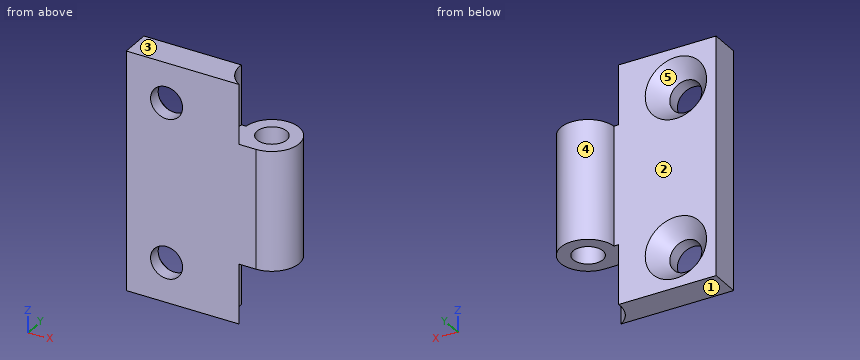
```python
from build123d import *

# Parameters (mm, degrees)
SKETCH1_R                                    = 2.38125
EXTRUDE1_DEPTH                               = 19.05
CUT_EXTRUDE1_DEPTH                           = 9.525
CSK_FOR_10_FLAT_HEAD_MACHINE_SCREW1_AT_COUNT = 2
CSK_FOR_10_FLAT_HEAD_MACHINE_SCREW1_AT_PITCH = 25.4


with BuildPart() as part:
    # Sketch1 → Extrude1 (new, symmetric)
    with BuildSketch(Plane.XY):
        with BuildLine():
            Line((-20.6375, 0), (0, 0))
            ThreePointArc((0, 0), (3.219925902, 1.417615701), (4.348688447, 4.7498))
            ThreePointArc((4.348688447, 4.7498), (0, 8.73125), (-4.348688447, 4.7498))
            Line((-4.348688447, 4.7498), (-20.6375, 4.7498))
            Line((-20.6375, 4.7498), (-20.6375, 0))
        make_face()
        with Locations(Location((0, 4.365625, 0), (0, 0, 180))):
            Circle(SKETCH1_R, mode=Mode.SUBTRACT)
    extrude(amount=EXTRUDE1_DEPTH, both=True)

    # Sketch2 → Cut-Extrude1 (cut)
    with BuildSketch(Plane.XY.offset(19.05)):
        with BuildLine():
            Line((-5.110688447, 4.7498), (-4.348688447, 4.7498))
            ThreePointArc((-4.348688447, 4.7498), (3.936533663, 7.969725902), (0, 0))
            Line((0, 0), (-2.684780288, 0))
            ThreePointArc((-2.684780288, 0), (-4.564261518, 2.034478581), (-5.110688447, 4.7498))
        make_face()
    cut_extrude1 = extrude(amount=-CUT_EXTRUDE1_DEPTH, mode=Mode.SUBTRACT)

    # Mirror1: Cut-Extrude1 across plane
    add(cut_extrude1.mirror(Plane.XY), mode=Mode.SUBTRACT)

    # Sketch6 → CSK for #10 Flat Head Machine Screw1 (revolve, cut)
    with BuildSketch(Plane(origin=(-14.224, 4.7498, -12.7), x_dir=(0, 0, 1), z_dir=(1, 0, 0))):
        Polygon((0, 0), (0, 4.7498), (2.5527, 4.7498), (2.5527, 2.688180894), (4.8895, 0), align=None)
    csk_for_10_flat_head_machine_screw1 = revolve(axis=Axis((-14.224, 11.0998, -12.7), (0, -1, 0)), mode=Mode.SUBTRACT)

    # CSK for #10 Flat Head Machine Screw1 at: CSK for #10 Flat Head Machine Screw1 ×2
    with Locations(*[(0, 0, i * CSK_FOR_10_FLAT_HEAD_MACHINE_SCREW1_AT_PITCH) for i in range(1, CSK_FOR_10_FLAT_HEAD_MACHINE_SCREW1_AT_COUNT)]):
        add(csk_for_10_flat_head_machine_screw1, mode=Mode.SUBTRACT)


solid = part.part
```
Could you check a few things on this model? Use its own coordinates, in mm. Face numbers are marked on the shaded views. A direction names the side the tool comes from. Round coordinates to 2 decimals unless told otherwise and drop trailing zeros. Loops run counter-clockwise (first coordinate to the right, second up) from the corner with the lowest first, then second, coordinate; pieces in that order, holes last. Notation, with made-up numbers: (0, -7) - (30, -7) arc R10 cw to (30, 10) - close; hole circle Ø2 at (-17.75, -30.75). An arc over 180 degrees is marked (long way). Answer in a Markdown table with one row per item. Add a question column.
(1) If we section it at D-D (y = 1.5): State how many separate pieces and enclosed holes the cut face has, plus the area to 3 significant figures.
(2) I'm going to push flat-ended pins straight in: pin 1 (6 mm diameter, centred on x = -14.224, z = -12.7, fed in from +Y); pin 2 (4 mm diameter, centred on x = -16, z = -1.5, fed in from +Y); pin 3 (3 mm diameter, centred on x = -3, z = 0, fed in from +Y). Where does each tip first touch, or does it pass through?
(3) If we section it at C-C (z = 6): Please give me the cut outline in (x, y), plus the area to 3 significant figures.
(4) For the marked faces 1 and 2, which set-ups out of +Z, -Z, +X, -X, +Y, -Y let a thin tool reach every point of the face, with its end or its side?
(5) I need wall thicknesses on line 1 along X through (y, z) = (4.25, -7.5); line 2 along Z through (x, y) = (-13.75, 3.25); line 3 along Z through (x, y) = (-2.5, 4.75) (3 decimals). Which ranges of each line are inside material? Lowest first, please.
(6) If we section it at B-B (y = 5.25): Please give me the cut outline in (x, z) (3 decimals).
(7) If we mould it in two halves opening along Z, with no side actions, what happens to the marked faces 3, 4 and 5? For each: pulls with the +Z half, pulls with the -Z half, needs draft (parallel to the pull), parting line crosses it, or undercut.
(8) If we section it at A-A (z = -12.7): Please give me the cut outline in (x, y), plus the area to 3 significant figures.
Model answer:
| question | item | result |
|---|---|---|
| 1 | separate pieces | 1 |
| 1 | enclosed holes | 2 |
| 1 | area | 727 mm² |
| 2 | pin 1 | stops at y = 2.58 |
| 2 | pin 2 | stops at y = 4.75 |
| 2 | pin 3 | stops at y = 8.47 |
| 3 | outline | (-20.64, 0) - (0, 0) arc R4.37 ccw (long way) to (-4.35, 4.75) - (-20.64, 4.75) - close; hole circle Ø4.76 at (0, 4.37) |
| 3 | area | 123 mm² |
| 4 | face 1 | -Z, +X, -X, +Y, -Y |
| 4 | face 2 | +Z, -Z, -X, +Y |
| 5 | line 1 | x = -20.64 to -2.38, 2.38 to 4.36 |
| 5 | line 2 | z = -19.05 to -16.25, -9.15 to 9.15, 16.25 to 19.05 |
| 5 | line 3 | z = -9.525 to 9.525 |
| 6 | outline | (-4.275, -9.525) - (-2.211, -9.525) - (-2.211, 9.525) - (-4.275, 9.525) - close; (2.211, -9.525) - (4.275, -9.525) - (4.275, 9.525) - (2.211, 9.525) - close |
| 7 | face 3 | pulls with the +Z half |
| 7 | face 4 | needs draft |
| 7 | face 5 | undercut |
| 8 | outline | (-20.64, 0) - (-16.78, 0) - (-16.78, 2.06) - (-19.11, 4.75) - (-20.64, 4.75) - close; (-11.67, 0) - (-2.68, 0) arc R5.13 cw to (-5.11, 4.75) - (-9.33, 4.75) - (-11.67, 2.06) - close |
| 8 | area | 46.3 mm² |
